Build history of the part. All positions in model axes, mm. A direction names the side the tool comes from. Round coordinates to 2 decimals unless told otherwise and drop trailing zeros. Write each loop counter-clockwise with the first axis right and the second up, starting at its lowest first coordinate (ties: lowest second). Pieces come first, ordered by that corner, then holes. Notation, with made-up numbers: (84.5, 42.25) -> (137.5, 42.25) arc R17 cw to (137.5, 58.25) -> close; hole circle Ø10 at (25.5, -38). An arc over 180 degrees is marked (long way). Answer as CSV lines item,"result".
from build123d import *

# Parameters (mm, degrees)
F0_W     = 152.4
F0_H     = 19.05
F1_DEPTH = 12.7
F2_R     = 27.294321
F3_DEPTH = 64.726328
F4_W     = 24.047904
F4_H     = 139.005154
F5_DEPTH = 25.4


with BuildPart() as f1:
    # F0 (on Front) → F1 (new body)
    with BuildSketch(Plane.XZ):
        Rectangle(F0_W, F0_H)
    extrude(amount=F1_DEPTH)

    # F2 (on face) → F3 (join)
    with BuildSketch(Plane.XY.offset(9.525)):
        with Locations((0, -16.311869)):
            Circle(F2_R)
    extrude(amount=F3_DEPTH)

    # F4 (on face) → F5 (join)
    with BuildSketch(Plane.XY.offset(74.251328)):
        with Locations((12.023952, -16.311869)):
            Rectangle(F4_W, F4_H)
        Polygon((24.047904, 53.190708), (24.047904, -85.814446), (48.095807, -85.814446), (48.095807, 124.323294), (0, 124.323294), (0, 53.190708), align=None)
        with Locations((-12.023952, -16.311869)):
            Rectangle(F4_W, F4_H)
    extrude(amount=F5_DEPTH)


solid = f1.part
1. Cut at A-A, the plane x = 44.5. Write the cut outline in (y, z) (3 decimals), then the cut area to 3 significant figures.
Results found:
outline,"(-85.814, 74.251) -> (124.323, 74.251) -> (124.323, 99.651) -> (-85.814, 99.651) -> close; (-12.7, -9.525) -> (0, -9.525) -> (0, 9.525) -> (-12.7, 9.525) -> close"
area,"5,580 mm2"
2. Probe line 1 along X through (y, z) = (52.5, 93); line 2 along Z through (x, y) = (3, 22.5); line 3 along X through (y, z) = (-17, 57.5). List the from-to ranges inside material, lowest first.
Results found:
line 1,"x = -24.05 to 48.1"
line 2,"z = 74.25 to 99.65"
line 3,"x = -27.29 to 27.29"
3. Mould opens along Z. For faces 1 (the flat face through (-1, -6, -9.525)), 2 (the flat face through (-1, -12.7, 0)), 3 (the flat face through (49, -6, 9.525)) say: +Z half, -Z half, draft (parallel to the pull), parting line (faces both ways), or undercut.
Results found:
face 1,"-Z half"
face 2,"draft"
face 3,"undercut"
4. Drop flat-ended pins along their axis: pin 1 Ø3.5 at (x, y) = (-7.5, 7.5) entering from -Z (3 decimals); pin 2 Ø1 at (x, y) = (-26, -19) entering from +Z; pin 3 Ø5.5 at (x, z) = (-25, -1.5) entering from -Y. Give the stop position or say it passes through.
Results found:
pin 1,"stops at z = 9.525"
pin 2,"stops at z = 74.25"
pin 3,"stops at y = -12.7"
5. Cut at C-C, the plane x = -37. Write the cut outline in (y, z) (3 decimals).
Results found:
outline,"(-12.7, -9.525) -> (0, -9.525) -> (0, 9.525) -> (-12.7, 9.525) -> close"
6. Cut at D-D, the plane y = 103. Write the cut outline in (x, z).
Results found:
outline,"(0, 74.25) -> (48.1, 74.25) -> (48.1, 99.65) -> (0, 99.65) -> close"
7. Cut at B-B, the plane z = 80.5. Write the cut outline in (x, y).
Results found:
outline,"(-24.05, -85.81) -> (48.1, -85.81) -> (48.1, 124.32) -> (0, 124.32) -> (0, 53.19) -> (-24.05, 53.19) -> close"
8. Which spindle directions (+Z, -Z, +X, -X, +Y, -Y) get a long thin tool onto all of the face, cutting with end or side? Do faces 4 (the flat face through (0, -25, 9.525)), 5 (the flat face through (12, 21, 99.651)), 6 (the flat face through (0, 89, 87)), 7 (the flat face through (0, 4, 9.525)), 8 (the flat face through (-24.048, -17, 87)). Say none if no direction does.
Results found:
face 4,"-Z, +X, -X, -Y"
face 5,"+Z, +X, -X, +Y, -Y"
face 6,"+Z, -Z, -X, +Y"
face 7,"-Z, +X, -X, +Y"
face 8,"+Z, -X, +Y, -Y"
